from build123d import *

# Parameters (mm, degrees)
F0_W     = 101.6
F0_H     = 101.6
F1_DEPTH = 76.2
F2_W     = 76.2
F2_H     = 76.2
F3_DEPTH = 63.5
F4_W     = 109.6
F4_H     = 109.6
F5_DEPTH = 81.28


with BuildPart() as f1:
    # F0 (on Top) → F1 (new body)
    with BuildSketch(Plane.XY):
        with Locations((50.8, 50.8)):
            Rectangle(F0_W, F0_H)
    extrude(amount=F1_DEPTH)

    # F2 (on face) → F3 (cut)
    with BuildSketch(Plane.XY.offset(76.2)):
        with Locations((50.8, 50.8)):
            Rectangle(F2_W, F2_H)
    extrude(amount=-F3_DEPTH, mode=Mode.SUBTRACT)


with BuildPart() as f5:
    # F4 (on Top) → F5 (new body)
    with BuildSketch(Plane.XY):
        with Locations((50.8, 50.8)):
            Rectangle(F4_W, F4_H)
    extrude(amount=F5_DEPTH)

    # F6: cut F1
    add(f1.part, mode=Mode.SUBTRACT)


solid = f5.part
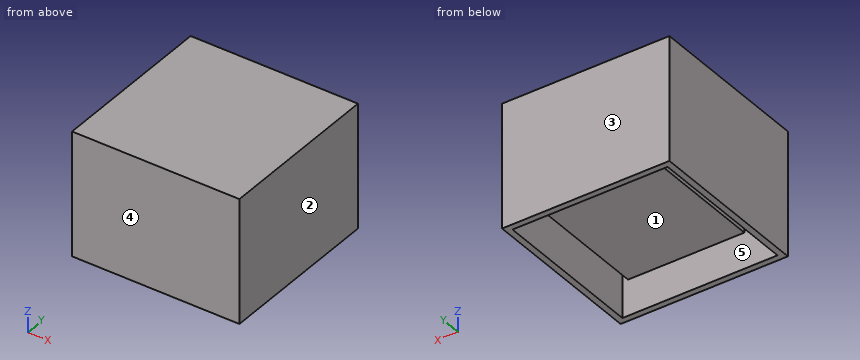
Source: CAD feature listing. Evaluate the final solid. Frame: model axes, mm. Face numbers are marked on the shaded views. A direction names the side the tool comes from. Give positions to 0.01 mm unless a question says otherwise; leave off trailing zeros. Loops run counter-clockwise (first coordinate to the right, second up) from the corner with the lowest first, then second, coordinate; pieces in that order, holes last. Notation, with made-up numbers: (58, -23) -> (106, -23) arc R22 ccw to (106, 15) -> close; hole circle Ø10 at (0, -27). An arc over 180 degrees is marked (long way). Use a Markdown table: item, result. Add a question column.
1) Section query A-A, the plane z = 52.5. Return the cut outline in (x, y).
2) Section query C-C, the plane z = 5.5. Return the cut outline in (x, y), then the cut area to 3 significant figures.
3) Section query B-B, the plane x = 90.5. Return the cut outline in (y, z).
4) Pull-direction query (X, two-part tool) for the marked faces 1, 2 and 3; classes: +X half, -X half, draft (parallel to the pull), parting line (faces both ways), or undercut.
5) Line query: line 1 along Y through (x, z) = (45.5, 34); line 2 along X through (y, z) = (6.5, 24.5). Output: solid intervals per line, ascending. Write a range as [from, to].
6) Reachability of the marked faces 4 and 5 from +Z, -Z, +X, -X, +Y, -Y: full face, straight path, thin tool, end or side. Return the list, or none.
7) First-contact query: pin 1 (1.5 mm diameter, centred on x = 13.5, y = 29, fed in from -Z). Flat tip, straight axial feed; report the tip coordinate or a pass-through.
Numbers:
| question | item | result |
|---|---|---|
| 1 | outline | (-4, -4) -> (105.6, -4) -> (105.6, 105.6) -> (-4, 105.6) -> close; (12.7, 12.7) -> (88.9, 12.7) -> (88.9, 88.9) -> (12.7, 88.9) -> close; hole (0, 0) -> (101.6, 0) -> (101.6, 101.6) -> (0, 101.6) -> close |
| 2 | outline | (-4, -4) -> (105.6, -4) -> (105.6, 105.6) -> (-4, 105.6) -> close; hole (0, 0) -> (101.6, 0) -> (101.6, 101.6) -> (0, 101.6) -> close |
| 2 | area | 1,690 mm2 |
| 3 | outline | (-4, 0) -> (0, 0) -> (0, 76.2) -> (101.6, 76.2) -> (101.6, 0) -> (105.6, 0) -> (105.6, 81.28) -> (-4, 81.28) -> close |
| 4 | face 1 | undercut |
| 4 | face 2 | +X half |
| 4 | face 3 | draft |
| 5 | line 1 | y = [-4, 0], [12.7, 88.9], [101.6, 105.6] |
| 5 | line 2 | x = [-4, 0], [101.6, 105.6] |
| 6 | face 4 | +Z, -Z, +X, -X, -Y |
| 6 | face 5 | -Z |
| 7 | pin 1 | stops at z = 12.7 |
